Input: part model. Units: mm. Frame: model coordinates. Coordinates: 2 decimals unless noted, no trailing zeros. Order: outer loops, then holes, each group sorted by start corner. A loop starts at its lowest first (then second) coordinate and runs counter-clockwise, first axis right, second up. Notation, with made-up numbers: (74.5, 7) - (107.5, 7) arc R17 ccw to (107.5, 15) - close; hole circle Ø3 at (43, -23.5). An arc over 180 degrees is marked (long way). Use a Markdown table: item, result. Add a question column.
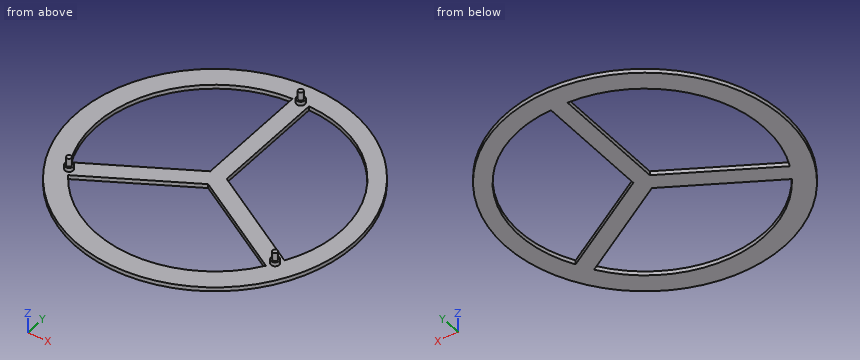
from build123d import *

# Parameters (mm, degrees)
SKETCH1_R           = 338.675134595
BOSS_EXTRUDE1_DEPTH = 10
SKETCH1_4_R         = 6
BOSS_EXTRUDE2_DEPTH = 40
SKETCH1_5_R         = 10
BOSS_EXTRUDE3_DEPTH = 20


with BuildPart() as part:
    # Sketch1 → Boss-Extrude1 (new body)
    with BuildSketch(Plane.XY):
        with Locations((-21.994465127, 277.22041187)):
            Circle(SKETCH1_R)
        with BuildLine():
            Line((-261.994465127, 115.562336497), (-21.994465127, 254.126401103))
            Line((-21.994465127, 254.126401103), (218.005534873, 115.562336497))
            ThreePointArc((218.005534873, 115.562336497), (-21.994465127, -12.146713653), (-261.994465127, 115.562336497))
        make_face(mode=Mode.SUBTRACT)
        with BuildLine():
            Line((-41.994465127, 565.895546465), (-41.994465127, 288.767417254))
            Line((-41.994465127, 288.767417254), (-281.994465127, 150.203352649))
            ThreePointArc((-281.994465127, 150.203352649), (-272.59374685, 421.903974632), (-41.994465127, 565.895546465))
        make_face(mode=Mode.SUBTRACT)
        with BuildLine():
            Line((238.005534873, 150.203352649), (-1.994465127, 288.767417254))
            Line((-1.994465127, 288.767417254), (-1.994465127, 565.895546465))
            ThreePointArc((-1.994465127, 565.895546465), (238.005534873, 427.33148186), (238.005534873, 150.203352649))
        make_face(mode=Mode.SUBTRACT)
    extrude(amount=BOSS_EXTRUDE1_DEPTH)

    # Sketch1<4> → Boss-Extrude2 (add)
    with BuildSketch(Plane.XY):
        with Locations((228.005534873, 132.882844573)):
            Circle(SKETCH1_4_R)
        with Locations((-271.994465127, 132.882844573)):
            Circle(SKETCH1_4_R)
        with Locations((-21.994465127, 565.895546465)):
            Circle(SKETCH1_4_R)
    extrude(amount=BOSS_EXTRUDE2_DEPTH)

    # Sketch1<5> → Boss-Extrude3 (add)
    with BuildSketch(Plane.XY):
        with Locations((-271.994465127, 132.882844573)):
            Circle(SKETCH1_5_R)
        with Locations((-21.994465127, 565.895546465)):
            Circle(SKETCH1_5_R)
        with Locations((228.005534873, 132.882844573)):
            Circle(SKETCH1_5_R)
    extrude(amount=BOSS_EXTRUDE3_DEPTH)


solid = part.part
1) Contact query for flat-ended pins moving along their axis: P1, Ø8, axis at x = 109.5, z = 5.5, coming from the +Y side; P2, Ø3, axis at y = 459, z = 3, coming from the +X side; P3, Ø8, axis at y = 441, z = 5, coming from the -X side. Output: stop coordinate, or through.
2) Material intervals for L1, parallel to X at y = 212, z = 5.5; L2, parallel to Y at x = 44, z = 8.5; L3, parallel to X at y = 273.5, z = 6.5, sorted ascending.
3) Cut plane A-A (x = -154.5). Return the cut outline in (y, z).
4) Cut plane C-C (y = 17). Return the cut outline in (x, z).
5) Cut plane D-D (z = 34). Return the cut outline in (x, y), and give its area (3 significant figures).
6) Cut plane B-B (y = 506.5). Return the cut outline in (x, z).
Computed:
| question | item | result |
|---|---|---|
| 1 | P1 | stops at y = 590.98 |
| 1 | P2 | stops at x = 264.71 |
| 1 | P3 | stops at x = -320.61 |
| 2 | L1 | x = -354.33 to -303.92, -174.96 to -94.96, 50.97 to 130.97, 264.29 to 310.34 |
| 2 | L2 | y = -54.96 to -4.52, 216.02 to 262.21, 562.05 to 609.4 |
| 2 | L3 | x = -360.65 to -311.34, -68.44 to 24.45, 274.71 to 316.66 |
| 3 | outline | (-34.46, 0) - (19.97, 0) - (19.97, 10) - (-34.46, 10) - close; (177.62, 0) - (223.81, 0) - (223.81, 10) - (177.62, 10) - close; (534.47, 0) - (588.9, 0) - (588.9, 10) - (534.47, 10) - close |
| 4 | outline | (-238.76, 0) - (-148.56, 0) - (-148.56, 10) - (-238.76, 10) - close; (104.57, 0) - (194.77, 0) - (194.77, 10) - (104.57, 10) - close |
| 5 | outline | circle Ø12 at (-271.99, 132.88); circle Ø12 at (-21.99, 565.9); circle Ø12 at (228.01, 132.88) |
| 5 | area | 339 mm2 |
| 6 | outline | (-271.26, 0) - (-198.53, 0) - (-198.53, 10) - (-271.26, 10) - close; (-41.99, 0) - (-1.99, 0) - (-1.99, 10) - (-41.99, 10) - close; (169.45, 0) - (227.27, 0) - (227.27, 10) - (169.45, 10) - close |
